Could you check a few things on this model? Use its own coordinates, in mm. Round coordinates to 2 decimals unless told otherwise and drop trailing zeros. Loops run counter-clockwise (first coordinate to the right, second up) from the corner with the lowest first, then second, coordinate; pieces in that order, holes last. Notation, with made-up numbers: M 56,31.25 L 66,31.25 A21 cw 66,64.25 Z; hole C 70,57 d4. An arc over 180 degrees is marked long. Answer in a Markdown table with one row per item.
```python
from build123d import *

# Parameters (mm, degrees)
BOSS_EXTRUDE1_DEPTH    = 3.175
FILLET1_R              = 2.54
SKETCH2_W              = 2.794
SKETCH2_H              = 38.1
CUT_EXTRUDE1_DEPTH     = 3.175
CUT_EXTRUDE2_START     = -3.175
CUT_EXTRUDE2_OUTLINE_W = 2.794
CUT_EXTRUDE2_OUTLINE_H = 35.802572731
CUT_EXTRUDE2_DEPTH     = 3.175
SKETCH4_W              = 2.794
SKETCH4_H              = 38.1
CUT_EXTRUDE3_DEPTH     = 3.175


# Read off the part's stored shape, not the designer's step: Cut-Extrude2
with BuildPart() as part:
    # Sketch1 → Boss-Extrude1 (new body)
    with BuildSketch(Plane.XY):
        Polygon((28.434847271, 23.464502165), (79.234847271, 23.464502165), (79.234847271, -36.860497835), (-123.965152729, -36.860497835), (-123.965152729, 23.464502165), (-73.165152729, 23.464502165), (-73.165152729, 83.789502165), (28.434847271, 83.789502165), align=None)
    extrude(amount=BOSS_EXTRUDE1_DEPTH)

    # Fillet1
    fillet1_edges = [part.edges().sort_by_distance(p)[0] for p in [
        (-123.965152729, 23.464502165, 1.5875),
        (-73.165152729, 23.464502165, 1.5875),
        (-73.165152729, 83.789502165, 1.5875),
        (28.434847271, 83.789502165, 1.5875),
        (28.434847271, 23.464502165, 1.5875),
        (79.234847271, 23.464502165, 1.5875),
        (79.234847271, -36.860497835, 1.5875),
        (-123.965152729, -36.860497835, 1.5875),
    ]]
    fillet(fillet1_edges, radius=FILLET1_R)

    # Sketch2 → Cut-Extrude1 (cut)
    with BuildSketch(Plane.XY.offset(3.175)):
        with Locations((15.925347271, 45.689502165)):
            Rectangle(SKETCH2_W, SKETCH2_H)
    extrude(amount=-CUT_EXTRUDE1_DEPTH, mode=Mode.SUBTRACT)

    # Cut-Extrude2 outline → Cut-Extrude2 (cut)
    with BuildSketch(Plane.XY.offset(3.175).offset(CUT_EXTRUDE2_START)):
        with Locations((-60.655652729, 46.8382158)):
            Rectangle(CUT_EXTRUDE2_OUTLINE_W, CUT_EXTRUDE2_OUTLINE_H)
    extrude(amount=CUT_EXTRUDE2_DEPTH, mode=Mode.SUBTRACT)

    # Sketch4 → Cut-Extrude3 (cut)
    with BuildSketch(Plane.XY.offset(3.175)):
        with Locations((-43.574152729, 46.047516436)):
            Rectangle(SKETCH4_W, SKETCH4_H)
    extrude(amount=-CUT_EXTRUDE3_DEPTH, mode=Mode.SUBTRACT)


solid = part.part
```
1) I want a section at B-B, the plane y = 34.5. Please give me the cut outline in (x, z) (3 decimals), plus the area to 3 significant figures.
Computed:
| item | result |
|---|---|
| outline | M -73.165,0 L -62.053,0 L -62.053,3.175 L -73.165,3.175 Z; M -59.259,0 L -44.971,0 L -44.971,3.175 L -59.259,3.175 Z; M -42.177,0 L 14.528,0 L 14.528,3.175 L -42.177,3.175 Z; M 17.322,0 L 28.435,0 L 28.435,3.175 L 17.322,3.175 Z |
| area | 296 mm² |
2) I want a section at A-A, the plane z = 1.15. Please give me the cut outline in (x, y), plus the area to 3 significant figures.
Computed:
| item | result |
|---|---|
| outline | M -123.97,-34.32 A2.54 ccw -121.43,-36.86 L 76.69,-36.86 A2.54 ccw 79.23,-34.32 L 79.23,20.92 A2.54 ccw 76.69,23.46 L 30.97,23.46 A2.54 cw 28.43,26 L 28.43,81.25 A2.54 ccw 25.89,83.79 L -70.63,83.79 A2.54 ccw -73.17,81.25 L -73.17,26 A2.54 cw -75.71,23.46 L -121.43,23.46 A2.54 ccw -123.97,20.92 Z; hole M -62.05,28.94 L -59.26,28.94 L -59.26,64.74 L -62.05,64.74 Z; hole M -44.97,27 L -42.18,27 L -42.18,65.1 L -44.97,65.1 Z; hole M 14.53,26.64 L 17.32,26.64 L 17.32,64.74 L 14.53,64.74 Z |
| area | 18,100 mm² |
3) I need wall thicknesses on line 1 (X direction, y = 49.5, z = 2.45); line 2 (X direction, y = 28.5, z = 2.15); line 3 (X direction, y = 21, z = 2.4). Which ranges of each line are inside material? Lowest first, please.
Computed:
| item | result |
|---|---|
| line 1 | x = -73.17 to -62.05, -59.26 to -44.97, -42.18 to 14.53, 17.32 to 28.43 |
| line 2 | x = -73.17 to -44.97, -42.18 to 14.53, 17.32 to 28.43 |
| line 3 | x = -123.96 to 79.23 |
4) I want a section at C-C, the plane x = -89. Please give me the cut outline in (y, z) (1 decimal).
Computed:
| item | result |
|---|---|
| outline | M -36.9,0 L 23.5,0 L 23.5,3.2 L -36.9,3.2 Z |
5) Will these pins go through, and if not, where does the flat tip stop? P1, Ø1, axis at x = 44.5, z = 1.5, coming from the +Y side; P2, Ø1.6, axis at y = 51, z = 1, coming from the -X side; P3, Ø1.6, axis at y = 39.5, z = 1, coming from the +X side.
Computed:
| item | result |
|---|---|
| P1 | stops at y = 23.46 |
| P2 | stops at x = -73.17 |
| P3 | stops at x = 28.43 |
